Here's how the part is built. I have some questions about the finished solid (model axes, mm). A direction names the side the tool comes from. Round coordinates to 2 decimals unless told otherwise and drop trailing zeros. Write each loop counter-clockwise with the first axis right and the second up, starting at its lowest first coordinate (ties: lowest second). Pieces come first, ordered by that corner, then holes. Notation, with made-up numbers: (38, 50.5) - (68, 50.5) arc R8 cw to (68, 63.5) - close; hole circle Ø11 at (-36.5, 81.5). An arc over 180 degrees is marked (long way). One line per question, with ' | ' between items. Start each with the question number.
(1) Will these pins go through, and if not, where does the flat tip stop? pin 1 (15 mm diameter, centred on x = 54.5, y = -228, fed in from -Z); pin 2 (9.5 mm diameter, centred on x = 58, y = -95, fed in from -Z); pin 3 (12 mm diameter, centred on y = -136, z = 65.5, fed in from -X).
(2) If I drill on L1, parallel to Z at x = 47.5, y = -108.5; L2, parallel to Y at x = 17.5, z = 8, over which ranges is the centre line in solid material (lowest first)?
(3) Imagine slicing it at B-B (x = 54). Write out the boundary of the cut face in (y, z), plus the area to 3 significant figures.
(4) Imagine slicing it at A-A (z = 59.5). Write out the boundary of the cut face in (x, y), plus the area to 3 significant figures.
(5) For faces 1 (the cylindrical face through (-70.746, -2.172, 6.261)), 2 (the flat face through (-13, -2, 12.7)), 3 (the flat face through (56, -221.456, 57)), 4 (the flat face through (56, -240.506, 64)), 5 (the flat face through (56, -231, 50.8)), which set-ups out of +Z, -Z, +X, -X, +Y, -Y let a thin tool reach every point of the face, with its end or its side?
(6) Imagine slicing it at C-C (y = -84). Write out the boundary of the cut face in (x, z).
(7) Imagine slicing it at D-D (z = 6). Write out the boundary of the cut face in (x, y) (3 decimals).
(8) Thinking about a two-plate mould opening in X: for faces 6 (the flat face through (46.727, -99, 66)), 7 (the flat face through (21, -11.906, 6)), 8 (the flat face through (65.777, -99, 64)), which applies, pulls with the +X half, pulls with the -X half, needs draft (parallel to the pull), parting line crosses it, or undercut?
from build123d import *

# Parameters (mm, degrees)
F0_W     = 19.0500000055
F0_H     = 19.05
F1_DEPTH = 12.7
F2_DEPTH = 76.2
F3_W     = 19.05
F3_H     = 209.55
F4_DEPTH = 12.7
F3_H_2   = 19.05
F5_DEPTH = 25.4


# Not quite as in the source:
# - a feature names something its author has since deleted; it is built from what else it names


with BuildPart() as f1:
    # F0 (on Top) → F1 (new body)
    with BuildSketch(Plane.XY):
        with BuildLine():
            Line((46.7271760769, 7.14375), (-61.2228239231, 7.14375))
            ThreePointArc((-61.2228239231, 7.14375), (-70.7478239286, -2.3812499973), (-61.2228239286, -11.90625))
            Line((-61.2228239286, -11.90625), (46.7271760714, -11.90625))
            Line((46.7271760714, -11.90625), (46.7271760769, 7.14375))
        make_face()
        with Locations((56.2521760742, -2.38125)):
            Rectangle(F0_W, F0_H)
    extrude(amount=F1_DEPTH)

    # F0 (on Top) → F2 (join)
    with BuildSketch(Plane.XY):
        with Locations((56.2521760742, -2.38125)):
            Rectangle(F0_W, F0_H)
    extrude(amount=F2_DEPTH)

    # F3 (on face) → F4 (join)
    with BuildSketch(Plane.XY.offset(76.2)):
        with Locations((56.2521760742, -116.68125)):
            Rectangle(F3_W, F3_H)
    extrude(amount=-F4_DEPTH)

    # F3 (on face) → F5 (join)
    with BuildSketch(Plane.XY.offset(76.2)):
        with Locations((56.2521760742, -230.98125)):
            Rectangle(F3_W, F3_H_2)
    extrude(amount=-F5_DEPTH)


with BuildPart() as f6_1:
    # F6: copy of F1
    add(f1.part)


solid = f1.part
Check sheet entries:
1) pin 1: z = 50.8 | pin 2: z = 63.5 | pin 3: x = 46.73
2) L1: 63.5 to 76.2 | L2: -11.91 to 7.14
3) outline: (-240.51, 50.8) - (-221.46, 50.8) - (-221.46, 63.5) - (-11.91, 63.5) - (-11.91, 0) - (7.14, 0) - (7.14, 76.2) - (-240.51, 76.2) - close | area: 4,600 mm^2
4) outline: (46.73, -240.51) - (65.78, -240.51) - (65.78, -221.46) - (46.73, -221.46) - close; (46.73, -11.91) - (65.78, -11.91) - (65.78, 7.14) - (46.73, 7.14) - close | area: 726 mm^2
5) face 1: +Z, -Z, -X | face 2: +Z, -X, +Y, -Y | face 3: -Z, +X, -X | face 4: +Z, -Z, +X, -X, -Y | face 5: -Z, +X, -X, -Y
6) outline: (46.73, 63.5) - (65.78, 63.5) - (65.78, 76.2) - (46.73, 76.2) - close
7) outline: (-61.223, -11.906) - (65.777, -11.906) - (65.777, 7.144) - (-61.223, 7.144) arc R9.525 ccw to start
8) face 6: pulls with the -X half | face 7: needs draft | face 8: pulls with the +X half
